Check sheet for the modelled part. Datum: model origin and axes. Units: mm. Face numbers are marked on the shaded views. A direction names the side the tool comes from. Give positions to 0.01 mm unless a question says otherwise; leave off trailing zeros. Write each loop counter-clockwise with the first axis right and the second up, starting at its lowest first coordinate (ties: lowest second). Pieces come first, ordered by that corner, then holes. Notation, with made-up numbers: M 54,34.5 L 87,34.5 A11 cw 87,38.5 Z; hole C 79,8.25 d5. An arc over 180 degrees is marked long. Use CSV: the item, a comma, the result in double quotes. Start each with the question number.
1. Cross-section at D-D, the plane z = 1.5. Enter the section's corners in (x, y).
2. Access from +Z, -Z, +X, -X, +Y, -Y to the whole of each face (thin tool, end or side, straight path). Record for the marked faces 1, 2 and 3.
3. Depth check by flat-ended pin: P1, Ø4, axis at y = 9, z = 13.5, coming from the +X side; P2, Ø5.5, axis at x = -12, y = 0.5, coming from the -Z side; P3, Ø5, axis at y = 14, z = 15.5, coming from the -X side. Enter the tip coordinate at first touch or a pass-through.
4. Cross-section at A-A, the plane z = 14.25. Enter the section's corners in (x, y), and give its area (3 significant figures).
5. Mould release check, pull along X, two halves, no side actions. Record for the marked faces 4, 5 and 6: +X half, -X half, draft (parallel to the pull), parting line (faces both ways), or undercut.
6. Scan lines: line 1 (Y direction, x = 0, z = 6.75); line 2 (X direction, y = -14.5, z = 10.25). Record each from-to range of solid material in increasing order.
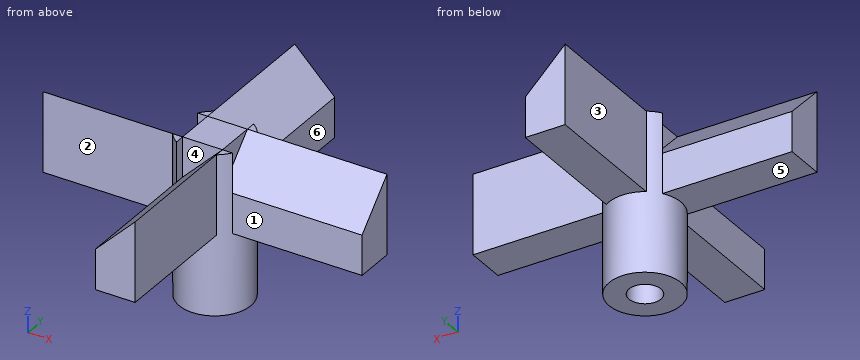
from build123d import *

# Parameters (mm, degrees)
F0_R     = 4.5
F1_DEPTH = 10
F2_W     = 5
F2_H     = 5
F3_DEPTH = 10
F4_SIZE  = 4.99999
F5_DEPTH = 10
F7_D     = 4
F7_DEPTH = 12
F7_TIP   = 1.2017212381


# Not quite as in the source:
# - a fillet or chamfer is up to 0.001 mm smaller than in the source, because OpenCascade refuses the exact size


with BuildPart() as f1:
    # F0 (on Top) → F1 (new body)
    with BuildSketch(Plane.XY):
        Circle(F0_R)
    extrude(amount=F1_DEPTH)

    # F2 (on face) → F3 (join)
    with BuildSketch(Plane.XY.offset(10)):
        with BuildLine():
            ThreePointArc((2.5, -3.7416573868), (0, -4.5), (-2.5, -3.7416573868))
            Line((-2.5, -3.7416573868), (-2.5, -20))
            Line((-2.5, -20), (2.5, -20))
            Line((2.5, -20), (2.5, -3.7416573868))
        make_face()
        with BuildLine():
            Line((-3.7416573868, 2.5), (-20, 2.5))
            Line((-20, 2.5), (-20, -2.5))
            Line((-20, -2.5), (-3.7416573868, -2.5))
            ThreePointArc((-3.7416573868, -2.5), (-4.5, 0), (-3.7416573868, 2.5))
        make_face()
        with BuildLine():
            Line((-2.5, 20), (-2.5, 3.7416573868))
            ThreePointArc((-2.5, 3.7416573868), (0, 4.5), (2.5, 3.7416573868))
            Line((2.5, 3.7416573868), (2.5, 20))
            Line((2.5, 20), (-2.5, 20))
        make_face()
        with BuildLine():
            Line((20, 2.5), (3.7416573868, 2.5))
            ThreePointArc((3.7416573868, 2.5), (4.3062430401, 1.3062430401), (4.5, 0))
            ThreePointArc((4.5, 0), (4.3062430401, -1.3062430401), (3.7416573868, -2.5))
            Line((3.7416573868, -2.5), (20, -2.5))
            Line((20, -2.5), (20, 2.5))
        make_face()
        with BuildLine():
            Line((3.7416573868, 2.5), (2.5, 2.5))
            Line((2.5, 2.5), (2.5, -2.5))
            Line((2.5, -2.5), (3.7416573868, -2.5))
            ThreePointArc((3.7416573868, -2.5), (4.3062430401, -1.3062430401), (4.5, 0))
            ThreePointArc((4.5, 0), (4.3062430401, 1.3062430401), (3.7416573868, 2.5))
        make_face()
        Rectangle(F2_W, F2_H)
        with BuildLine():
            Line((2.5, -2.5), (-2.5, -2.5))
            Line((-2.5, -2.5), (-2.5, -3.7416573868))
            ThreePointArc((-2.5, -3.7416573868), (0, -4.5), (2.5, -3.7416573868))
            Line((2.5, -3.7416573868), (2.5, -2.5))
        make_face()
        with BuildLine():
            Line((-2.5, 2.5), (-3.7416573868, 2.5))
            ThreePointArc((-3.7416573868, 2.5), (-4.5, 0), (-3.7416573868, -2.5))
            Line((-3.7416573868, -2.5), (-2.5, -2.5))
            Line((-2.5, -2.5), (-2.5, 2.5))
        make_face()
        with BuildLine():
            Line((-2.5, 3.7416573868), (-2.5, 2.5))
            Line((-2.5, 2.5), (2.5, 2.5))
            Line((2.5, 2.5), (2.5, 3.7416573868))
            ThreePointArc((2.5, 3.7416573868), (0, 4.5), (-2.5, 3.7416573868))
        make_face()
    extrude(amount=F3_DEPTH)

    # F4 (size 5 in the source; OpenCascade refuses exactly that, so slightly less here)
    f4_edges = [f1.edges().sort_by_distance(p)[0] for p in [
        (-2.5, -11.25, 20),
        (-11.25, 2.5, 20),
        (2.5, 11.25, 20),
        (11.25, -2.5, 20),
    ]]
    chamfer(f4_edges, length=F4_SIZE)

    # F5 (add): faces of the model
    f5_faces = [f1.faces().sort_by_distance(p)[0] for p in [
        (-2.940797231, 2.940797231, 10),
        (2.940797231, 2.940797231, 10),
        (2.940797231, -2.940797231, 10),
        (-2.940797231, -2.940797231, 10),
    ]]
    extrude(f5_faces, amount=F5_DEPTH)

    # F7
    with Locations(Plane(origin=(0, 0, 0), x_dir=(1, 0, 0), z_dir=(0, 0, -1))):
        with Locations((0, 0)):
            Hole(F7_D / 2, depth=F7_DEPTH)
            with Locations((0, 0, -(F7_DEPTH + F7_TIP / 2))):  # 118° drill point
                Cone(0, F7_D / 2, F7_TIP, mode=Mode.SUBTRACT)


solid = f1.part
Worked answers:
1,outline,"C 0,0 d9; hole C 0,0 d4"
2,face 1,"+Z, -Z, +X, -Y"
2,face 2,"+Z, -Z, -X, -Y"
2,face 3,"+Z, -Z, -X, +Y"
3,P1,"stops at x = 2.5"
3,P2,"stops at z = 10"
3,P3,"stops at x = -2.5"
4,outline,"M -20,-2.5 L -3.74,-2.5 A4.5 ccw -2.5,-3.74 L -2.5,-20 L 2.5,-20 L 2.5,-3.74 A4.5 ccw 3.74,-2.5 L 20,-2.5 L 20,2.5 L 3.74,2.5 A4.5 ccw 2.5,3.74 L 2.5,20 L -2.5,20 L -2.5,3.74 A4.5 ccw -3.74,2.5 L -20,2.5 Z"
4,area,"378 mm^2"
5,face 4,"undercut"
5,face 5,"draft"
5,face 6,"+X half"
6,line 1,"y = -4.5 to -2, 2 to 4.5"
6,line 2,"x = -2.5 to 2.5"
